Can you work these out from the model? Positions are in its coordinate system, mm. A direction names the side the tool comes from. Give positions to 0.01 mm unless a question says otherwise; leave off trailing zeros. Write each loop counter-clockwise with the first axis right and the second up, starting at its lowest first coordinate (ties: lowest second). Pieces come first, ordered by that corner, then holes. Notation, with made-up numbers: M -11.5,4 L 21.5,4 A26 ccw 21.5,42 Z; hole C 23,-5 d3. An arc over 180 degrees is marked long. Answer as CSV lines item,"result". Start each with the question number.
```python
from build123d import *

# Parameters (mm, degrees)
SKETCH3_R           = 14
SKETCH3_R_2         = 1.75
SKETCH3_R_3         = 4
BOSS_EXTRUDE1_DEPTH = 2
BOSS_EXTRUDE2_START = 50
SKETCH4_R           = 14
SKETCH4_R_2         = 12.65
BOSS_EXTRUDE2_DEPTH = 50
BOSS_EXTRUDE3_START = -52
SKETCH5_R           = 3
BOSS_EXTRUDE3_DEPTH = 52
SKETCH6_R           = 13.15
CUT_EXTRUDE1_DEPTH  = 50
SKETCH8_R           = 3.2
SKETCH8_R_2         = 3
CUT_EXTRUDE2_DEPTH  = 52


with BuildPart() as part:
    # Sketch3 → Boss-Extrude1 (new body)
    with BuildSketch(Plane.XY):
        Circle(SKETCH3_R)
        with Locations((8.5, 0)):
            Circle(SKETCH3_R_2, mode=Mode.SUBTRACT)
        with Locations((-8.5, 0)):
            Circle(SKETCH3_R_2, mode=Mode.SUBTRACT)
        Circle(SKETCH3_R_3, mode=Mode.SUBTRACT)
    extrude(amount=BOSS_EXTRUDE1_DEPTH)

    # Sketch4 → Boss-Extrude2 (add)
    with BuildSketch(Plane(origin=(0, 0, 0), x_dir=(-1, 0, 0), z_dir=(0, 0, -1)).offset(BOSS_EXTRUDE2_START)):
        Circle(SKETCH4_R)
        Circle(SKETCH4_R_2, mode=Mode.SUBTRACT)
    extrude(amount=-BOSS_EXTRUDE2_DEPTH)

    # Sketch5 → Boss-Extrude3 (add)
    # profile 1 of 4: a face of its own
    with BuildSketch(Plane.XY.offset(2).offset(BOSS_EXTRUDE3_START)):
        with BuildLine():
            Line((24.720866981, -28.352755346), (13.218427546, 4.612285031))
            ThreePointArc((13.218427546, 4.612285031), (13.803224001, 2.339018422), (14, 0))
            ThreePointArc((14, 0), (-2.339018422, -13.803224001), (-13.218427546, 4.612285031))
            Line((-13.218427546, 4.612285031), (-24.720866981, -28.352755346))
            ThreePointArc((-24.720866981, -28.352755346), (-23.047527639, -26.036090908), (-20.378622129, -25.014356081))
            Line((-20.378622129, -25.014356081), (-14.656053545, -8.613947671))
            ThreePointArc((-14.656053545, -8.613947671), (0, -17), (14.656053545, -8.613947671))
            Line((14.656053545, -8.613947671), (20.378622129, -25.014356081))
            ThreePointArc((20.378622129, -25.014356081), (23.047527639, -26.036090908), (24.720866981, -28.352755346))
        make_face()
    # profile 2 of 4: a face of its own
    with BuildSketch(Plane.XY.offset(2).offset(BOSS_EXTRUDE3_START)):
        with BuildLine():
            Line((5.004377394, -23.279258169), (16.663748404, -33.724167731))
            ThreePointArc((16.663748404, -33.724167731), (15.168880977, -31.288522016), (15.252243256, -28.431941997))
            Line((15.252243256, -28.431941997), (7.006128352, -21.044757531))
            ThreePointArc((7.006128352, -21.044757531), (0, -18.365509765), (-7.006128352, -21.044757531))
            Line((-7.006128352, -21.044757531), (-15.252243256, -28.431941997))
            ThreePointArc((-15.252243256, -28.431941997), (-15.063463577, -29.205891607), (-15, -30))
            ThreePointArc((-15, -30), (-15.434846225, -32.039453606), (-16.663748404, -33.724167731))
            Line((-16.663748404, -33.724167731), (-5.004377394, -23.279258169))
            ThreePointArc((-5.004377394, -23.279258169), (0, -21.365509765), (5.004377394, -23.279258169))
        make_face()
    # profile 3 of 4: a face of its own
    with BuildSketch(Plane.XY.offset(2).offset(BOSS_EXTRUDE3_START)):
        with BuildLine():
            ThreePointArc((-20.378622129, -25.014356081), (-23.047527639, -26.036090908), (-24.720866981, -28.352755346))
            ThreePointArc((-24.720866981, -28.352755346), (-22.773500981, -34.160251472), (-16.663748404, -33.724167731))
            ThreePointArc((-16.663748404, -33.724167731), (-15.434846225, -32.039453606), (-15, -30))
            ThreePointArc((-15, -30), (-15.063463577, -29.205891607), (-15.252243256, -28.431941997))
            ThreePointArc((-15.252243256, -28.431941997), (-17.226499019, -25.839748528), (-20.378622129, -25.014356081))
        make_face()
        with Locations((-20, -30)):
            Circle(SKETCH5_R, mode=Mode.SUBTRACT)
    # profile 4 of 4: a face of its own
    with BuildSketch(Plane.XY.offset(2).offset(BOSS_EXTRUDE3_START)):
        with BuildLine():
            ThreePointArc((25, -30), (24.929722858, -29.164636278), (24.720866981, -28.352755346))
            ThreePointArc((24.720866981, -28.352755346), (23.047527639, -26.036090908), (20.378622129, -25.014356081))
            ThreePointArc((20.378622129, -25.014356081), (17.226499019, -25.839748528), (15.252243256, -28.431941997))
            ThreePointArc((15.252243256, -28.431941997), (15.168880977, -31.288522016), (16.663748404, -33.724167731))
            ThreePointArc((16.663748404, -33.724167731), (22.039453606, -34.565153775), (25, -30))
        make_face()
        with Locations((20, -30)):
            Circle(SKETCH5_R, mode=Mode.SUBTRACT)
    extrude(amount=BOSS_EXTRUDE3_DEPTH)

    # Sketch6 → Cut-Extrude1 (cut)
    with BuildSketch(Plane(origin=(0, 0, -50), x_dir=(-1, 0, 0), z_dir=(0, 0, -1))):
        Circle(SKETCH6_R)
    extrude(amount=-CUT_EXTRUDE1_DEPTH, mode=Mode.SUBTRACT)

    # Sketch8 → Cut-Extrude2 (cut)
    # profile 1 of 4: a face of its own
    with BuildSketch(Plane(origin=(0, 0, -50), x_dir=(-1, 0, 0), z_dir=(0, 0, -1))):
        with Locations((20, -30)):
            Circle(SKETCH8_R)
        with Locations((20, -30)):
            Circle(SKETCH8_R_2, mode=Mode.SUBTRACT)
    # profile 2 of 4: a face of its own
    with BuildSketch(Plane(origin=(0, 0, -50), x_dir=(-1, 0, 0), z_dir=(0, 0, -1))):
        with Locations((-20, -30)):
            Circle(SKETCH8_R)
        with Locations((-20, -30)):
            Circle(SKETCH8_R_2, mode=Mode.SUBTRACT)
    # profile 3 of 4: a face of its own
    with BuildSketch(Plane(origin=(0, 0, -50), x_dir=(-1, 0, 0), z_dir=(0, 0, -1))):
        with Locations((20, -30)):
            Circle(SKETCH8_R_2)
    # profile 4 of 4: a face of its own
    with BuildSketch(Plane(origin=(0, 0, -50), x_dir=(-1, 0, 0), z_dir=(0, 0, -1))):
        with Locations((-20, -30)):
            Circle(SKETCH8_R_2)
    extrude(amount=-CUT_EXTRUDE2_DEPTH, mode=Mode.SUBTRACT)


solid = part.part
```
1) I want a section at B-B, the plane y = 0. Please give me the cut outline in (x, z).
2) I want a section at D-D, the plane y = -10.5. Please give me the cut outline in (x, z).
3) I'm going to push flat-ended pins straight in: P1, Ø4, axis at x = -7.5, z = -9.5, coming from the +Y side; P2, Ø2, axis at x = 6, z = -35.5, coming from the +Y side; P3, Ø8, axis at x = 13, z = -6, coming from the +Y side. Where does each tip first touch, or does it pass through?
4) Thinking about a two-plate mould opening in X: for faces 5 (the flat face through (-18.89, -11.64, -24.36)), 6 (the flat face through (-11.071, -24.687, -24.364)), 7 (the flat face through (11.2, -24.8, -24.4)), 8 (the flat face through (0, -10, 2)), which applies, released by +X, released by -X, zero draft, split by the parting line, or undercut?
5) I want a section at C-C, the plane x = -8.5. Please give me the cut outline in (y, z), then the cut area to 3 significant figures.
6) I want a section at A-A, the plane z = -45. Please give me the cut outline in (x, y), then the cut area to 3 significant figures.
7) On a 3-axis mill with a long thin cutter (end or side, diameter ignored), from which of +Z, -Z, +X, -X, +Y, -Y can I reach the whole of each face in a straight line? I mean faces 1 (the flat face through (3, 3, 0)), 2 (the cylindrical face through (0, 14, -24)), 3 (the flat face through (-10.916, -28.575, -24.364)), 4 (the flat face through (17.477, -16.699, -24.364)). Say none if no direction works.
8) I need wall thicknesses on L1, parallel to X at y = -10, z = -23; L2, parallel to Y at x = -9, z = -36; L3, parallel to Y at x = 2.5, z = -0.5. Which ranges of each line are inside material? Lowest first, please. Write a range as from..to.
Values found:
1,outline,"M -14.83,-50 L -13.15,-50 L -13.15,0 L -10.25,0 L -10.25,2 L -14.83,2 Z; M -6.75,0 L -4,0 L -4,2 L -6.75,2 Z; M 4,0 L 6.75,0 L 6.75,2 L 4,2 Z; M 10.25,0 L 13.15,0 L 13.15,-50 L 14.83,-50 L 14.83,2 L 10.25,2 Z"
2,outline,"M -18.49,-50 L -15.31,-50 L -15.31,2 L -18.49,2 Z; M -13.37,-50 L -7.92,-50 L -7.92,0 L 7.92,0 L 7.92,-50 L 13.37,-50 L 13.37,2 L -13.37,2 Z; M 15.31,-50 L 18.49,-50 L 18.49,2 L 15.31,2 Z"
3,P1,"stops at y = 12.87"
3,P2,"stops at y = 13.08"
3,P3,"stops at y = 10.72"
4,face 5,"released by -X"
4,face 6,"undercut"
4,face 7,"undercut"
4,face 8,"zero draft"
5,outline,"M -26.41,-50 L -22.38,-50 L -22.38,2 L -26.41,2 Z; M -14.72,-50 L -10.03,-50 L -10.03,0 L -1.75,0 L -1.75,2 L -14.72,2 Z; M 1.75,0 L 10.03,0 L 10.03,-50 L 11.12,-50 L 11.12,2 L 1.75,2 Z"
5,area,"543 mm²"
6,outline,"M -24.72,-28.35 A5 ccw -16.66,-33.72 L -5,-23.28 A7.5 cw 5,-23.28 L 16.66,-33.72 A5 ccw 24.72,-28.35 L 13.22,4.61 A14 ccw -13.22,4.61 Z; hole C -20,-30 d6.4; hole M -20.38,-25.01 A5 cw -15.25,-28.43 L -7.01,-21.04 A10.5 cw 7.01,-21.04 L 15.25,-28.43 A5 cw 20.38,-25.01 L 14.66,-8.61 A17 cw -14.66,-8.61 Z; hole C 0,0 d26.3; hole C 20,-30 d6.4"
6,area,"538 mm²"
7,face 1,"-Z"
7,face 2,"+Z, -Z, +Y"
7,face 3,"+Z, -Z, -Y"
7,face 4,"+Z, -Z"
8,L1,"x = -18.32..-15.14, -13.75..-8.54, 8.54..13.75, 15.14..18.32"
8,L2,"y = -26.86..-22.83, -14.42..-9.59, 9.59..10.72"
8,L3,"y = -21.79..-18.67, -16.82..-12.91, 12.91..13.77"
